from build123d import *

# Parameters (mm, degrees)
SKETCH1_W           = 88
SKETCH1_H           = 88
BOSS_EXTRUDE1_DEPTH = 18
FILLET1_R           = 10
SKETCH2_R           = 2.15
CUT_EXTRUDE1_DEPTH  = 19
SKETCH5_R           = 4
CUT_EXTRUDE4_DEPTH  = 13
SKETCH6_R           = 4.25
CUT_EXTRUDE5_DEPTH  = 40
CHAMFER1_SIZE       = 20
CHAMFER1_SIZE2      = 0.349101299
SKETCH7_R           = 24
CUT_EXTRUDE6_DEPTH  = 19
FILLET2_R           = 10


with BuildPart() as part:
    # Sketch1 → Boss-Extrude1 (new body)
    with BuildSketch(Plane(origin=(0, 0, 0), x_dir=(1, 0, 0), z_dir=(0, 1, 0))):
        Rectangle(SKETCH1_W, SKETCH1_H)
    extrude(amount=BOSS_EXTRUDE1_DEPTH)

    # Fillet1
    fillet1_edges = [part.edges().sort_by_distance(p)[0] for p in [
        (-44, 9, -44),
        (-44, 9, 44),
        (44, 9, 44),
        (44, 9, -44),
    ]]
    fillet(fillet1_edges, radius=FILLET1_R)

    # Sketch2 → Cut-Extrude1 (cut, through all)
    with BuildSketch(Plane(origin=(0, 18, 0), x_dir=(1, 0, 0), z_dir=(0, 1, 0))):
        with Locations((-34, 34)):
            Circle(SKETCH2_R)
        with Locations((34, 34)):
            Circle(SKETCH2_R)
        with Locations((34, -34)):
            Circle(SKETCH2_R)
        with Locations((-34, -34)):
            Circle(SKETCH2_R)
    extrude(amount=-CUT_EXTRUDE1_DEPTH, mode=Mode.SUBTRACT)

    # Sketch5 → Cut-Extrude4 (cut)
    with BuildSketch(Plane(origin=(0, 18, 0), x_dir=(1, 0, 0), z_dir=(0, 1, 0))):
        with Locations((-34, 34)):
            Circle(SKETCH5_R)
        with Locations((34, 34)):
            Circle(SKETCH5_R)
        with Locations((34, -34)):
            Circle(SKETCH5_R)
        with Locations((-34, -34)):
            Circle(SKETCH5_R)
    extrude(amount=-CUT_EXTRUDE4_DEPTH, mode=Mode.SUBTRACT)

    # Sketch6 → Cut-Extrude5 (cut)
    with BuildSketch(Plane.XY.offset(44)):
        with Locations((0, 9)):
            Circle(SKETCH6_R)
    extrude(amount=-CUT_EXTRUDE5_DEPTH, mode=Mode.SUBTRACT)

    # Chamfer1
    chamfer1_edges = [part.edges().sort_by_distance(p)[0] for p in [
        (-4.25, 9, 4),
    ]]
    chamfer1_side = [part.faces().sort_by_distance(p)[0] for p in [
        (-4.25, 9, 24),
    ]]
    chamfer(chamfer1_edges, length=CHAMFER1_SIZE, length2=CHAMFER1_SIZE2, reference=chamfer1_side[0])

    # Sketch7 → Cut-Extrude6 (cut, through all)
    with BuildSketch(Plane(origin=(0, 18, 0), x_dir=(1, 0, 0), z_dir=(0, 1, 0))):
        with Locations((-44, 0)):
            Circle(SKETCH7_R)
        with Locations((44, 0)):
            Circle(SKETCH7_R)
    extrude(amount=-CUT_EXTRUDE6_DEPTH, mode=Mode.SUBTRACT)

    # Fillet2
    fillet2_edges = [part.edges().sort_by_distance(p)[0] for p in [
        (-44, 9, 24),
        (-44, 9, -24),
        (44, 9, 24),
        (44, 9, -24),
    ]]
    fillet(fillet2_edges, radius=FILLET2_R)


solid = part.part
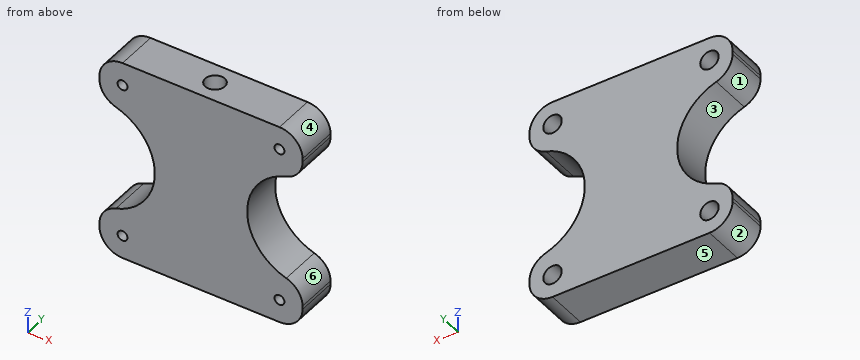
Verification items for the finished model (mm, model axes). Face numbers are marked on the shaded views. A direction names the side the tool comes from. Give positions to 0.01 mm unless a question says otherwise; leave off trailing zeros. Loops run counter-clockwise (first coordinate to the right, second up) from the corner with the lowest first, then second, coordinate; pieces in that order, holes last. Notation, with made-up numbers: (-3.5, -23) - (14.5, -23) arc R15 ccw to (14.5, -19) - close; hole circle Ø3 at (-33, 89). An arc over 180 degrees is marked (long way). Write item = value, one per line. Start each with the question number.
Q1. Cross-section at A-A, the plane y = 3.25. Enter the section's corners in (x, z), and give its area (3 significant figures).
Q2. Mould release check, pull along Z, two halves, no side actions. Record for the marked faces 1, 2, 3 and 4: released by +Z, released by -Z, zero draft, split by the parting line, or undercut.
Q3. Tool access check on the marked faces 5 and 6. Record the directions out of +Z, -Z, +X, -X, +Y, -Y that give a thin tool (end or side, any length) a straight path to the whole face; none if there is none.
Q4. Cross-section at B-B, the plane x = 25. Enter the section's corners in (y, z).
Q5. Thickness scan on line 1 (X direction, y = 14.25, z = 34); line 2 (X direction, y = 3.75, z = -34); line 3 (X direction, y = 12.75, z = 34). Record the ranges inside material, lowest first.
Q6. Cross-section at C-C, the plane z = 11. Enter the section's corners in (x, y), and give its area (3 significant figures).
Q7. Cross-section at D-D, the plane y = 16.5. Enter the section's corners in (x, z).
Q8. Depth check by flat-ended pin: P1, Ø4, axis at x = -34, z = 34, coming from the -Y side; P2, Ø2, axis at y = 14, z = 5.5, coming from the -X side; P3, Ø5, axis at x = 34, z = -34, coming from the +Y side; P4, Ø1, axis at y = 14, z = 31, coming from the -X side. Enter the tip coordinate at first touch or a pass-through.
Answer key:
q1.outline = (-44, -34) arc R10 ccw to (-34, -44) - (34, -44) arc R10 ccw to (44, -34) - (44, -32.5) arc R10 ccw to (36.94, -22.94) arc R24 cw to (36.94, 22.94) arc R10 ccw to (44, 32.5) - (44, 34) arc R10 ccw to (34, 44) - (-34, 44) arc R10 ccw to (-44, 34) - (-44, 32.5) arc R10 ccw to (-36.94, 22.94) arc R24 cw to (-36.94, -22.94) arc R10 ccw to (-44, -32.5) - close; hole circle Ø4.3 at (-34, -34); hole circle Ø4.3 at (-34, 34); hole circle Ø4.3 at (34, -34); hole circle Ø4.3 at (34, 34)
q1.area = 5,740 mm^2
q2.face_1 = undercut
q2.face_2 = released by -Z
q2.face_3 = undercut
q2.face_4 = released by +Z
q3.face_5 = -Z, +X, -X, +Y, -Y
q3.face_6 = +X, +Y, -Y
q4.outline = (0, -44) - (18, -44) - (18, -14.66) - (0, -14.66) - close; (0, 14.66) - (18, 14.66) - (18, 44) - (0, 44) - close
q5.line_1 = -44 to -38, -30 to 30, 38 to 44
q5.line_2 = -44 to -36.15, -31.85 to 31.85, 36.15 to 44
q5.line_3 = -44 to -38, -30 to -2, 2 to 30, 38 to 44
q6.outline = (-22.67, 0) - (22.67, 0) - (22.67, 18) - (-22.67, 18) - close; hole circle Ø8.05 at (0, 9)
q6.area = 765 mm^2
q7.outline = (-44, -34) arc R10 ccw to (-34, -44) - (34, -44) arc R10 ccw to (44, -34) - (44, -32.5) arc R10 ccw to (36.94, -22.94) arc R24 cw to (36.94, 22.94) arc R10 ccw to (44, 32.5) - (44, 34) arc R10 ccw to (34, 44) - (-34, 44) arc R10 ccw to (-44, 34) - (-44, 32.5) arc R10 ccw to (-36.94, 22.94) arc R24 cw to (-36.94, -22.94) arc R10 ccw to (-44, -32.5) - close; hole circle Ø8 at (-34, -34); hole circle Ø8 at (-34, 34); hole circle Ø8 at (34, -34); hole circle Ø8 at (34, 34)
q8.P1 = through
q8.P2 = -20.9
q8.P3 = 5
q8.P4 = -43.95
